```python
from build123d import *

# Parameters (mm, degrees)
CROQUIS1_R                 = 30
SALIENTE_EXTRUIR1_DEPTH    = 50
CROQUIS3_R                 = 24.13
CORTAR_EXTRUIR1_DEPTH      = 15
CORTAR_EXTRUIR2_START      = -85
CROQUIS3_2_R               = 24.13
CORTAR_EXTRUIR2_DEPTH      = 15
CROQUIS4_R                 = 30
CROQUIS4_R_2               = 24.13
CORTAR_EXTRUIR3_DEPTH      = 32.5
CROQUIS5_R                 = 24.13
SALIENTE_EXTRUIR2_DEPTH    = 50
CROQUIS6_R                 = 30
SALIENTE_EXTRUIR3_DEPTH    = 17.8
CORTAR_EXTRUIR4_START      = -15
CROQUIS7_R                 = 24.13
CORTAR_EXTRUIR4_DEPTH      = 15
CROQUIS9_R                 = 20
CORTAR_EXTRUIR5_DEPTH      = 104.07764064
REDONDEO1_R                = 2
CORTAR_EXTRUIR6_REACH      = 89.321
CORTAR_EXTRUIR6_END_RADIUS = 20
CROQUIS10_R                = 20


with BuildPart() as part:
    # Croquis1 → Saliente-Extruir1 (new, symmetric)
    with BuildSketch(Plane(origin=(0, 0, 0), x_dir=(1, 0, 0), z_dir=(0, 1, 0))):
        with Locations(Location((0, 0, 0), (0, 0, 90))):
            Circle(CROQUIS1_R)
    extrude(amount=SALIENTE_EXTRUIR1_DEPTH, both=True)

    # Croquis3 → Cortar-Extruir1 (cut)
    with BuildSketch(Plane(origin=(0, 50, 0), x_dir=(1, 0, 0), z_dir=(0, 1, 0))):
        with Locations(Location((0, 0, 0), (0, 0, 270))):
            Circle(CROQUIS3_R)
    extrude(amount=-CORTAR_EXTRUIR1_DEPTH, mode=Mode.SUBTRACT)

    # Croquis3<2> → Cortar-Extruir2 (cut)
    with BuildSketch(Plane(origin=(0, 50, 0), x_dir=(1, 0, 0), z_dir=(0, 1, 0)).offset(CORTAR_EXTRUIR2_START)):
        with Locations(Location((0, 0, 0), (0, 0, 270))):
            Circle(CROQUIS3_2_R)
    extrude(amount=-CORTAR_EXTRUIR2_DEPTH, mode=Mode.SUBTRACT)

    # Croquis4 → Cortar-Extruir3 (cut, symmetric)
    with BuildSketch(Plane(origin=(0, 0, 0), x_dir=(1, 0, 0), z_dir=(0, 1, 0))):
        with Locations(Location((0, 0, 0), (0, 0, 90))):
            Circle(CROQUIS4_R)
        with Locations(Location((0, 0, 0), (0, 0, 270))):
            Circle(CROQUIS4_R_2, mode=Mode.SUBTRACT)
    extrude(amount=CORTAR_EXTRUIR3_DEPTH, both=True, mode=Mode.SUBTRACT)

    # Croquis5 → Saliente-Extruir2 (add)
    with BuildSketch(Plane(origin=(0, 0, 0), x_dir=(0, 0, -1), z_dir=(1, 0, 0))):
        Circle(CROQUIS5_R)
    extrude(amount=SALIENTE_EXTRUIR2_DEPTH)

    # Croquis6 → Saliente-Extruir3 (add)
    with BuildSketch(Plane(origin=(50, 0, 0), x_dir=(0, 0, -1), z_dir=(1, 0, 0))):
        Circle(CROQUIS6_R)
    extrude(amount=-SALIENTE_EXTRUIR3_DEPTH)

    # Croquis7 → Cortar-Extruir4 (cut)
    with BuildSketch(Plane(origin=(50, 0, 0), x_dir=(0, 0, -1), z_dir=(1, 0, 0)).offset(CORTAR_EXTRUIR4_START)):
        Circle(CROQUIS7_R)
    extrude(amount=CORTAR_EXTRUIR4_DEPTH, mode=Mode.SUBTRACT)

    # Croquis9 → Cortar-Extruir5 (cut, through all)
    with BuildSketch(Plane.XZ.offset(35)):
        with Locations(Location((0, 0, 0), (0, 0, 270))):
            Circle(CROQUIS9_R)
    extrude(amount=-CORTAR_EXTRUIR5_DEPTH, mode=Mode.SUBTRACT)

    # Redondeo1
    redondeo1_edges = [part.edges().sort_by_distance(p)[0] for p in [
        (15.589160136, -15.589160136, -18.418332885),
        (24.13, 24.13, 2.6592e-05),
    ]]
    fillet(redondeo1_edges, radius=REDONDEO1_R)

    # Cortar-Extruir6: up to this cylinder (the profile starts outside it)
    cortar_extruir6_end = Plane(origin=(0, 0, 0), z_dir=(0, -1, 0)) * Cylinder(CORTAR_EXTRUIR6_END_RADIUS, 219.642, mode=Mode.PRIVATE)
    # Croquis10 → Cortar-Extruir6 (cut, up to the surface)
    with BuildSketch(Plane(origin=(35, 0, 0), x_dir=(0, 0, -1), z_dir=(1, 0, 0)), mode=Mode.PRIVATE) as cortar_extruir6_sk1:
        Circle(CROQUIS10_R)
    cortar_extruir6_tool1 = extrude(cortar_extruir6_sk1.sketch, amount=-CORTAR_EXTRUIR6_REACH, mode=Mode.PRIVATE) - cortar_extruir6_end
    add(cortar_extruir6_tool1.solids().sort_by_distance((35, 0, 0))[0], mode=Mode.SUBTRACT)


solid = part.part
```
Build history of the part. All positions in model axes, mm. A direction names the side the tool comes from. Coordinates: 2 decimals unless noted, no trailing zeros. Write each loop counter-clockwise with the first axis right and the second up, starting at its lowest first coordinate (ties: lowest second). Pieces come first, ordered by that corner, then holes.
1. Pull direction Z, two halves, no side cores. Call faces 4 (the cylindrical face through (23.03, 16.308, 17.785)), 5 (the flat face through (50, 25, -2)), 6 (the flat face through (20, 35, 3)): released by +Z, released by -Z, zero draft, split by the parting line, or undercut.
Answer block:
face 4: split by the parting line
face 5: zero draft
face 6: undercut
2. Drill centre lines: probe 1 along Y at (x, z) = (23.5, 0); probe 2 along Y at (x, z) = (5, -24.5); probe 3 along X at (y, z) = (27.5, -2.5). Where is each one in solid material? Low to high.
Answer block:
probe 1: y = -35 to -20, 20 to 35
probe 2: y = -50 to -32.5, 32.5 to 50
probe 3: x = -24 to -19.84, 19.84 to 24, 32.2 to 50
3. Drop flat-ended pins along their axis: pin 1 (24 mm diameter, centred on y = -3.5, z = -11.5, fed in from +X); pin 2 (24 mm diameter, centred on x = -6, z = -0.5, fed in from +Y); pin 3 (3 mm diameter, centred on y = -1.5, z = -15.5, fed in from -X); pin 4 (8 mm diameter, centred on y = 18.5, z = 20, fed in from -X). Give the stop position or say it passes through.
Answer block:
pin 1: stops at x = 35
pin 2: passes through
pin 3: stops at x = -19.65
pin 4: stops at x = -18.06
4. Band-saw the part on B-B, the plane x = 41. Give the cut face in (y, z).
Answer block:
outline: circle Ø60 at (0, 0); hole circle Ø48.26 at (0, 0)
5. 3-axis set-ups, long thin cutter, end or side, ignore diameter. For faces 1 (the flat face through (-25, -32.5, -2)), 2 (the cylindrical face through (-1.32, 41.37, 29.97)), 3 (the cylindrical face through (42.395, 7.248, -23.016)): which of +Z, -Z, +X, -X, +Y, -Y reach the whole face in a straight line?
Answer block:
face 1: none
face 2: +Y
face 3: +X
6. Band-saw the part on A-A, the plane z = 0. Give the number of separate pieces and of enclosed holes in the cut face, and give its area (3 significant figures).
Answer block:
separate pieces: 3
enclosed holes: 0
area: 1,120 mm2
